Here's how the part is built. I have some questions about the finished solid (model axes, mm). A direction names the side the tool comes from. Round coordinates to 2 decimals unless told otherwise and drop trailing zeros. Write each loop counter-clockwise with the first axis right and the second up, starting at its lowest first coordinate (ties: lowest second). Pieces come first, ordered by that corner, then holes. Notation, with made-up numbers: (52, -25) - (106, -25) arc R7 cw to (106, -14) - close; hole circle Ø3 at (38.5, -18.75). An arc over 180 degrees is marked (long way). One line per item, written item: value. Start each with the question number.
Item 1: Imagine slicing it at A-A, the plane y = -9. Please give me the cut outline in (x, z).
Item 2: Imagine slicing it at D-D, the plane x = 26. Please give me the cut outline in (y, z).
Item 3: If I drill on line 1 (Y direction, x = 0, z = -0.5); line 2 (Y direction, x = 20.5, z = -1.95); line 3 (X direction, y = -4, z = -0.2), over which ranges is the centre line in solid material (lowest first)?
Item 4: Thinking about a two-plate mould opening in X: for faces 1 (the face through (0, 0, -3.5)), 2 (the face through (20.356, 5.328, -0.352)), which applies, released by +X, released by -X, zero draft, split by the parting line, or undercut?
Item 5: Imagine slicing it at C-C, the plane y = 22. Please give me the cut outline in (x, z), then the cut area to 3 significant figures.
Item 6: For P1, Ø14.5, axis at x = 0, y = 18, coming from the +Z side; P2, Ø3, axis at y = 14.5, z = -1, coming from the -X side; P3, Ø3, axis at y = -19, z = -3, coming from the +X side, each with a flat end and sliding along its axis, tell me the tip position at first contact or that it passes through.
Item 7: Imagine slicing it at B-B, the plane z = 1.65. Count the separate pieces of the cut face and the enclosed holes in it, then the cut area to 3 significant figures.
Item 8: For faces 3 (the face through (-23.37, 5.61, -0.35)), 4 (the face through (16, -9, -2.5)), which set-ups out of +Z, -Z, +X, -X, +Y, -Y let a thin tool reach every point of the face, with its end or its side?
```python
from build123d import *

# Parameters (mm, degrees)
SKETCH1_R           = 30
SKETCH1_R_2         = 8
BOSS_EXTRUDE1_DEPTH = 2.5
SKETCH3_R           = 30
BOSS_EXTRUDE2_DEPTH = 1
CIRPATTERN1_COUNT   = 3
CIRPATTERN2_COUNT   = 12


with BuildPart() as part:
    # Sketch1 → Boss-Extrude1 (new, symmetric)
    with BuildSketch(Plane.XY):
        Circle(SKETCH1_R)
        with Locations((0, 18)):
            Circle(SKETCH1_R_2, mode=Mode.SUBTRACT)
        with Locations((15.588457268, -9)):
            Circle(SKETCH1_R_2, mode=Mode.SUBTRACT)
        with Locations((-15.588457268, -9)):
            Circle(SKETCH1_R_2, mode=Mode.SUBTRACT)
    extrude(amount=BOSS_EXTRUDE1_DEPTH, both=True)

    # Sketch3 → Boss-Extrude2 (add)
    with BuildSketch(Plane(origin=(0, 0, -2.5), x_dir=(-1, 0, 0), z_dir=(0, 0, -1))):
        Circle(SKETCH3_R)
    extrude(amount=BOSS_EXTRUDE2_DEPTH)

    # Sketch6 → M4x0.7 Tapped Hole1 (revolve, cut)
    with BuildSketch(Plane(origin=(-21.733331092, 5.823428515, -3.5), x_dir=(0, 1, 0), z_dir=(1, 0, 0))):
        Polygon((0, 0), (0, 11.091420021), (1.65, 10.1), (1.65, 0.375), (2.025, 0), align=None)
    m4x0_7_tapped_hole1 = revolve(axis=Axis((-21.733331092, 5.823428515, -9.85), (0, 0, 1)), mode=Mode.SUBTRACT)

    # Sketch8 → M4x0.7 Tapped Hole2 (revolve, cut)
    with BuildSketch(Plane(origin=(-15.155444566, 8.75, -3.5), x_dir=(0, 1, 0), z_dir=(1, 0, 0))):
        Polygon((0, 0), (0, 11.091420021), (1.65, 10.1), (1.65, 0.375), (2.025, 0), align=None)
    m4x0_7_tapped_hole2 = revolve(axis=Axis((-15.155444566, 8.75, -9.85), (0, 0, 1)), mode=Mode.SUBTRACT)

    # CirPattern1: M4x0.7 Tapped Hole2 ×3 about axis
    cirpattern1_axis = Axis((0.169620148, -0.06701082, 0), (0, 0, 1))
    for i in range(1, CIRPATTERN1_COUNT):
        add(m4x0_7_tapped_hole2.rotate(cirpattern1_axis, i * 360 / CIRPATTERN1_COUNT), mode=Mode.SUBTRACT)

    # CirPattern2: M4x0.7 Tapped Hole1 ×12 about axis, 6 skipped
    cirpattern2_axis = Axis((0.098499141, -0.026092579, 0), (0, 0, -1))
    add([m4x0_7_tapped_hole1.rotate(cirpattern2_axis, i * 360 / CIRPATTERN2_COUNT) for i in range(1, CIRPATTERN2_COUNT) if i not in (2, 3, 6, 7, 10, 11)], mode=Mode.SUBTRACT)


solid = part.part
```
Values follow:
1. outline: (-28.62, -3.5) - (28.62, -3.5) - (28.62, 2.5) - (23.59, 2.5) - (23.59, -2.5) - (7.59, -2.5) - (7.59, 2.5) - (-7.59, 2.5) - (-7.59, -2.5) - (-23.59, -2.5) - (-23.59, 2.5) - (-28.62, 2.5) - close
2. outline: (-14.97, -3.5) - (14.97, -3.5) - (14.97, 2.5) - (-14.97, 2.5) - close
3. line 1: y = -30 to -19.39, -16.11 to 10, 26 to 30
3. line 2: y = -21.9 to -15.31, -2.69 to 5, 6.65 to 21.9
3. line 3: x = -29.73 to -21.83, -9.34 to 9.34, 21.83 to 29.73
4. face 1: zero draft
4. face 2: undercut
5. outline: (-20.4, -3.5) - (20.4, -3.5) - (20.4, 2.5) - (6.93, 2.5) - (6.93, -2.5) - (-6.93, -2.5) - (-6.93, 2.5) - (-20.4, 2.5) - close
5. area: 175 mm^2
6. P1: stops at z = -2.5
6. P2: stops at x = -27.04
6. P3: stops at x = 24.37
7. separate pieces: 1
7. enclosed holes: 12
7. area: 2,150 mm^2
8. face 3: +Z, -Z
8. face 4: +Z
